Here's the drawing with two shaded views (mm, measured from the low corner). I have some questions. A direction names the side the tool comes from. Round coordinates to 2 decimals unless told otherwise and drop trailing zeros. Write each loop counter-clockwise with the first axis right and the second up, starting at its lowest first coordinate (ties: lowest second). Pieces come first, ordered by that corner, then holes. Notation, with made-up numbers: M -15,86 L 18,86 A19 ccw 18,109 Z; hole C -39,-9.5 d4. An arc over 180 degrees is marked long. Answer as a JSON object with one key per item and string values. Group by question number.
1) I'm going to push flat-ended pins straight in: pin 1 Ø2.5 at (x, z) = (46, 46) entering from -Y; pin 2 Ø2.5 at (x, y) = (23, 4) entering from -Z; pin 3 Ø2.5 at (y, z) = (5, 24) entering from -X. Where does each tip first touch, or does it pass through?
2) Suppose I cut it at D-D, the plane z = 30.5. Write out the boundary of the cut face in (x, y), and give its area (3 significant figures).
3) Suppose I cut it at C-C, the plane y = 4.5. Write out the boundary of the cut face in (x, z).
4) Suppose I cut it at A-A, the plane x = 46. Write out the boundary of the cut face in (y, z), and give its area (3 significant figures).
5) Please list where these lines run through material, in increasing order: L1, parallel to X at y = 0.5, z = 46; L2, parallel to Z at x = 12.5, y = 1.5. Write a range as [from, to].
6) On a 3-axis mill with a long thin cutter (end or side, diameter ignored), from which of +Z, -Z, +X, -X, +Y, -Y can I reach the whole of each face in a straight line? I mean the marked faces 1 and 2. Say none if no direction works.
7) If we mould it in two halves opening along X, with no side actions, what happens to the marked faces 3, 4 and 5? For each: +X half, -X half, draft (parallel to the pull), parting line (faces both ways), or undercut.
8) Suppose I cut it at B-B, the plane z = 46. Write out the boundary of the cut face in (x, y), and give its area (3 significant figures).
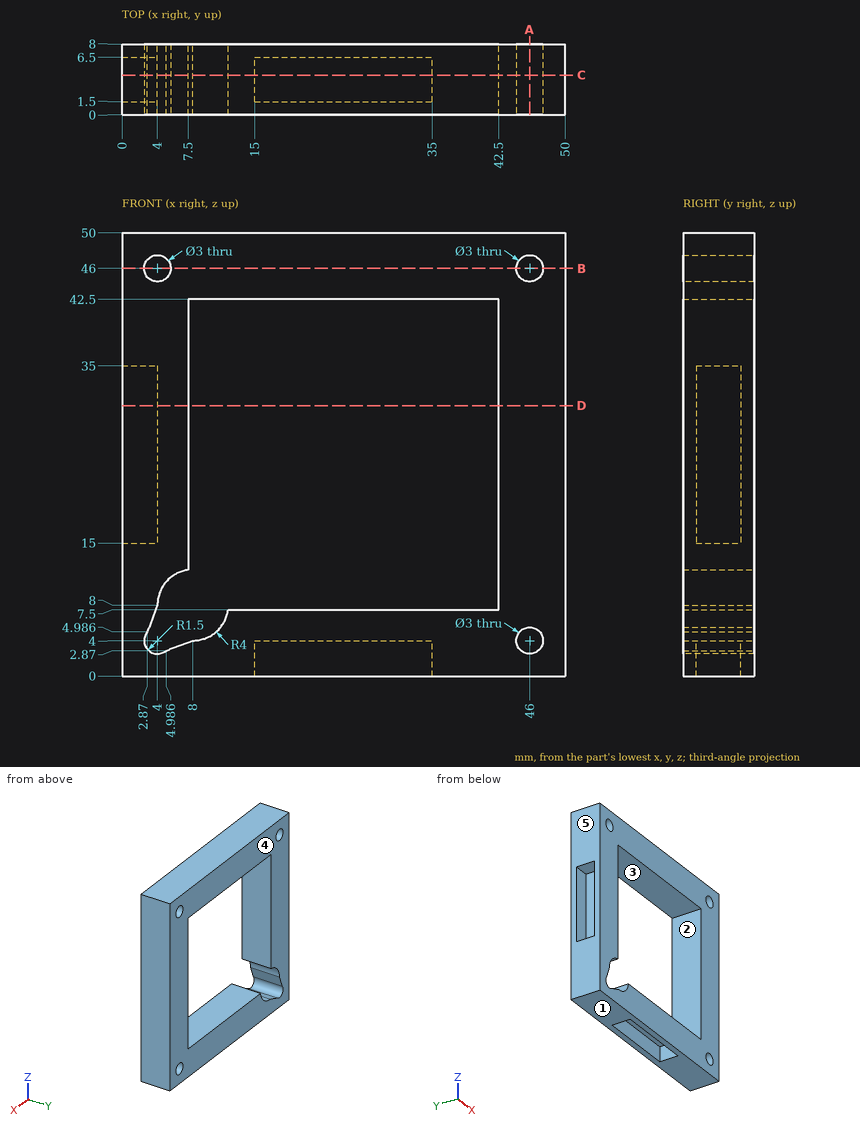
Results:
{
 "1": {"pin 1": "through", "pin 2": "z = 4", "pin 3": "x = 4"},
 "2": {"outline": "M 0,0 L 7.5,0 L 7.5,8 L 0,8 L 0,6.5 L 4,6.5 L 4,1.5 L 0,1.5 Z; M 42.5,0 L 50,0 L 50,8 L 42.5,8 Z", "area": "100 mm^2"},
 "3": {"outline": "M 0,0 L 15,0 L 15,4 L 35,4 L 35,0 L 50,0 L 50,50 L 0,50 L 0,35 L 4,35 L 4,15 L 0,15 Z; hole C 4,46 d3; hole M 2.87,4.99 A1.5 ccw 4.99,2.87 L 8,4 A4 ccw 11.97,7.5 L 42.5,7.5 L 42.5,42.5 L 7.5,42.5 L 7.5,11.97 A4 ccw 4,8 Z; hole C 46,4 d3; hole C 46,46 d3"},
 "4": {"outline": "M 0,0 L 8,0 L 8,2.5 L 0,2.5 Z; M 0,5.5 L 8,5.5 L 8,44.5 L 0,44.5 Z; M 0,47.5 L 8,47.5 L 8,50 L 0,50 Z", "area": "352 mm^2"},
 "5": {"L1": "[0, 2.5], [5.5, 44.5], [47.5, 50]", "L2": "[0, 7.5], [42.5, 50]"},
 "6": {"face 1": "-Z, +X, -X, +Y, -Y", "face 2": "+Y, -Y"},
 "7": {"face 3": "undercut", "face 4": "draft", "face 5": "-X half"},
 "8": {"outline": "M 0,0 L 2.5,0 L 2.5,8 L 0,8 Z; M 5.5,0 L 44.5,0 L 44.5,8 L 5.5,8 Z; M 47.5,0 L 50,0 L 50,8 L 47.5,8 Z", "area": "352 mm^2"}
}
